from build123d import *

# Parameters (mm, degrees)
SKETCH1_R           = 1.25
BOSS_EXTRUDE1_DEPTH = 2
FILLET1_R           = 2.5


with BuildPart() as part:
    # Sketch1 → Boss-Extrude1 (new body)
    with BuildSketch(Plane(origin=(0, 0, 0), x_dir=(1, 0, 0), z_dir=(0, 1, 0))):
        with BuildLine():
            Line((-103.965757813, 67.162425071), (-33.817700106, 107.662425071))
            Line((-33.817700106, 107.662425071), (-14.010882201, 73.356010123))
            ThreePointArc((-14.010882201, 73.356010123), (-9.775048525, 74.210673935), (-8.39729226, 70.115002459))
            Line((-8.39729226, 70.115002459), (31.216343551, 70.115002459))
            Line((31.216343551, 70.115002459), (31.216343551, -10.884997541))
            Line((31.216343551, -10.884997541), (-8.39729226, -10.884997541))
            ThreePointArc((-8.39729226, -10.884997541), (-9.775048525, -14.980669016), (-14.010882201, -14.126005204))
            Line((-14.010882201, -14.126005204), (-33.817700106, -48.432420153))
            Line((-33.817700106, -48.432420153), (-103.965757813, -7.932420153))
            Line((-103.965757813, -7.932420153), (-84.158939907, 26.373994796))
            ThreePointArc((-84.158939907, 26.373994796), (-87.017017318, 29.615002459), (-84.158939907, 32.856010123))
            Line((-84.158939907, 32.856010123), (-103.965757813, 67.162425071))
        make_face()
        with Locations(Location((-83.75035682, 29.615002459, 0), (0, 0, 270))):
            Circle(SKETCH1_R, mode=Mode.SUBTRACT)
        with Locations(Location((-11.408378774, 71.381662958, 0), (0, 0, 270))):
            Circle(SKETCH1_R, mode=Mode.SUBTRACT)
        with Locations(Location((-11.408378774, -12.151658039, 0), (0, 0, 270))):
            Circle(SKETCH1_R, mode=Mode.SUBTRACT)
    extrude(amount=BOSS_EXTRUDE1_DEPTH)

    # Fillet1
    fillet1_edges = [part.edges().sort_by_distance(p)[0] for p in [
        (-14.010882201, 1, -73.356010123),
        (-8.39729226, 1, -70.115002459),
        (-8.39729226, 1, 10.884997541),
        (-14.010882201, 1, 14.126005204),
        (-84.158939907, 1, -26.373994796),
        (-84.158939907, 1, -32.856010123),
    ]]
    fillet(fillet1_edges, radius=FILLET1_R)


solid = part.part
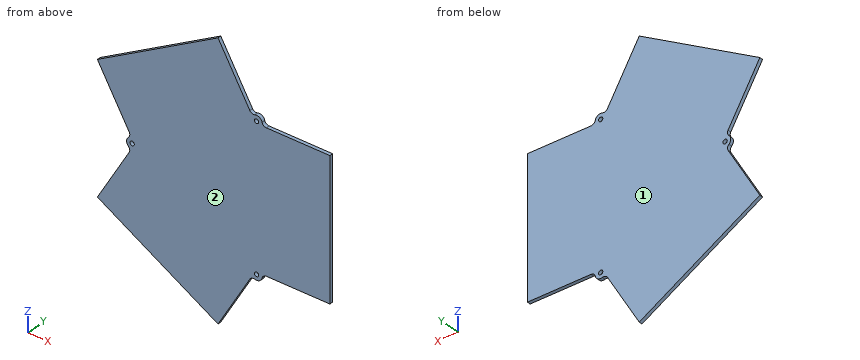
Could you check a few things on this model? Use its own coordinates, in mm. Face numbers are marked on the shaded views. Coordinates: 2 decimals unless noted, no trailing zeros. Loops run counter-clockwise (first coordinate to the right, second up) from the corner with the lowest first, then second, coordinate; pieces in that order, holes last. Notation, with made-up numbers: (-26, 48) -> (23, 48) arc R24 cw to (23, 72) -> close; hole circle Ø4 at (62.5, -3). An arc over 180 degrees is marked (long way). Answer in a Markdown table with one row per item.
(1) Imagine slicing it at B-B (z = -7). List the corners of the cut face in (x, y) for me, plus the area to 3 significant figures.
Results found:
| item | result |
|---|---|
| outline | (-95.34, 0) -> (31.22, 0) -> (31.22, 2) -> (-95.34, 2) -> close |
| area | 253 mm^2 |
(2) Imagine slicing it at A-A (y = 1). List the corners of the cut face in (x, z) for me (3 decimals), plus the area to 3 significant figures.
Results found:
| item | result |
|---|---|
| outline | (-103.966, -67.162) -> (-33.818, -107.662) -> (-15.322, -75.627) arc R2.5 cw to (-12.399, -74.495) arc R3.267 ccw to (-8.217, -72.08) arc R2.5 cw to (-5.775, -70.115) -> (31.216, -70.115) -> (31.216, 10.885) -> (-5.775, 10.885) arc R2.5 cw to (-8.217, 12.85) arc R3.267 ccw to (-12.399, 15.265) arc R2.5 cw to (-15.322, 16.397) -> (-33.818, 48.432) -> (-103.966, 7.932) -> (-85.47, -24.103) arc R2.5 cw to (-85.951, -27.201) arc R3.267 ccw to (-85.951, -32.029) arc R2.5 cw to (-85.47, -35.127) -> close; hole circle Ø2.5 at (-83.75, -29.615); hole circle Ø2.5 at (-11.408, -71.382); hole circle Ø2.5 at (-11.408, 12.152) |
| area | 13,400 mm^2 |
(3) If I drill on probe 1 along Z at (x, y) = (0.5, 0.6) (3 decimals); probe 2 along Z at (x, y) = (-41, 0.15); probe 3 along X at (y, z) = (1.05, -21), over which ranges is the centre line in solid material (lowest first)?
Results found:
| item | result |
|---|---|
| probe 1 | z = -70.115 to 10.885 |
| probe 2 | z = -103.52 to 44.29 |
| probe 3 | x = -87.26 to 31.22 |
(4) Will these pins go through, and if not, where does the flat tip stop? pin 1 Ø1.5 at (x, z) = (-11.41, -71.38) entering from -Y; pin 2 Ø6 at (x, z) = (-25, 31) entering from -Y; pin 3 Ø1 at (x, y) = (13.5, 0.5) entering from +Z (3 decimals).
Results found:
| item | result |
|---|---|
| pin 1 | passes through |
| pin 2 | stops at y = 0 |
| pin 3 | stops at z = 10.885 |
(5) Thinking about a two-plate mould opening in Y: for the marked faces 1 and 2, which applies, released by +Y, released by -Y, zero draft, split by the parting line, or undercut?
Results found:
| item | result |
|---|---|
| face 1 | released by +Y |
| face 2 | released by -Y |
(6) Imagine slicing it at C-C (x = -36). List the corners of the cut face in (y, z) for me, plus the area to 3 significant figures.
Results found:
| item | result |
|---|---|
| outline | (0, -106.4) -> (2, -106.4) -> (2, 47.17) -> (0, 47.17) -> close |
| area | 307 mm^2 |
